Design review of the part shown in the three views and the two pictorial views. Dimensions are in mm from the part's minimum x, y and z. A direction names the side the tool comes from. Round coordinates to 2 decimals unless told otherwise and drop trailing zeros. Loops run counter-clockwise (first coordinate to the right, second up) from the corner with the lowest first, then second, coordinate; pieces in that order, holes last.
1. To check wall thickness, follow line 1 along Z through (x, y) = (70.9, 5.5); line 2 along X through (y, z) = (24, 48.5); line 3 along Y through (x, z) = (71, 6.5). State the ranges of each line that lie inside material, in increasing order.
2. Consider section B-B on y = 30. State the section outline as (x, z) points, then the cut area to 3 significant figures.
3. Clearance check with flat-ended pins moving along their axes: pin 1 Ø5 at (y, z) = (29.5, 33) entering from -X; pin 2 Ø1.5 at (y, z) = (9, 29.5) entering from -X; pin 3 Ø1.5 at (x, z) = (70.5, 19.5) entering from +Y; pin 4 Ø8 at (x, y) = (98.5, 8.5) entering from +Z. State where each tip first meets the part, or that it passes through.
4. Draft analysis for pull direction X (two halves, no side actions). For the marked faces 1, 2, 3 and 4, state which applies: released by +X, released by -X, zero draft, split by the parting line, or undercut.
5. Consider section D-D on x = 70. State the section outline as (y, z) points.
6. Consider section C-C on z = 27. State the section outline as (x, y) points, then the cut area to 3 significant figures.
7. Tool access review of the marked faces 5, 6, 7 and 8: name each direction out of +Z, -Z, +X, -X, +Y, -Y from which nothing blocks a thin tool from reaching the whole face with its end or side.
8. Consider section A-A on x = 13. State the section outline as (y, z) points.
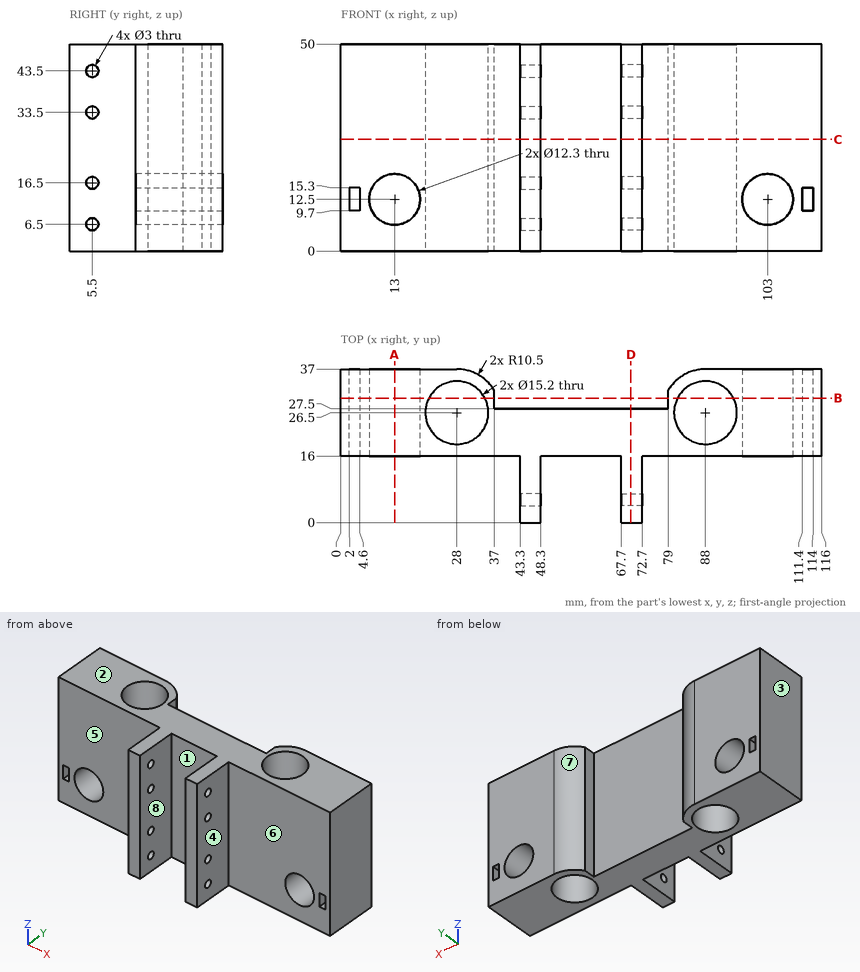
Resolved:
1. line 1: z = 0 to 5, 8 to 15, 18 to 32, 35 to 42, 45 to 50
1. line 2: x = 0 to 20.82, 35.18 to 80.82, 95.18 to 116
1. line 3: y = 0 to 4, 7 to 27.5
2. outline: (0, 0) - (21.25, 0) - (21.25, 50) - (0, 50) - close; (34.75, 0) - (37, 0) - (37, 50) - (34.75, 50) - close; (79, 0) - (81.25, 0) - (81.25, 50) - (79, 50) - close; (94.75, 0) - (116, 0) - (116, 50) - (94.75, 50) - close; hole (2, 9.7) - (4.6, 9.7) - (4.6, 15.3) - (2, 15.3) - close; hole circle Ø12.3 at (13, 12.5); hole circle Ø12.3 at (103, 12.5); hole (111.4, 9.7) - (114, 9.7) - (114, 15.3) - (111.4, 15.3) - close
2. area: 2,080 mm2
3. pin 1: stops at x = 0
3. pin 2: stops at x = 43.3
3. pin 3: stops at y = 27.5
3. pin 4: passes through
4. face 1: undercut
4. face 2: zero draft
4. face 3: released by -X
4. face 4: released by +X
5. outline: (0, 0) - (27.5, 0) - (27.5, 50) - (0, 50) - close; hole circle Ø3 at (5.5, 6.5); hole circle Ø3 at (5.5, 16.5); hole circle Ø3 at (5.5, 33.5); hole circle Ø3 at (5.5, 43.5)
6. outline: (0, 16) - (43.3, 16) - (43.3, 0) - (48.3, 0) - (48.3, 16) - (67.7, 16) - (67.7, 0) - (72.7, 0) - (72.7, 16) - (116, 16) - (116, 37) - (88, 37) arc R10.5 ccw to (79, 31.91) - (79, 27.5) - (37, 27.5) - (37, 31.91) arc R10.5 ccw to (28, 37) - (0, 37) - close; hole circle Ø15.2 at (28, 26.5); hole circle Ø15.2 at (88, 26.5)
6. area: 1,810 mm2
7. face 5: +Z, -Z, -X, -Y
7. face 6: +Z, -Z, +X, -Y
7. face 7: +Z, -Z, +Y
7. face 8: +Z, -Z, -Y
8. outline: (16, 0) - (37, 0) - (37, 6.35) - (16, 6.35) - close; (16, 18.65) - (37, 18.65) - (37, 50) - (16, 50) - close
